For this review, take the finished solid that the model builds, in its own axes (mm). Face numbers are marked on the shaded views. A direction names the side the tool comes from. Give positions to 0.01 mm unless a question says otherwise; leave off trailing zeros. Write each loop counter-clockwise with the first axis right and the second up, starting at its lowest first coordinate (ties: lowest second). Pieces come first, ordered by that corner, then holes. Notation, with made-up numbers: M -26.75,-36.5 L 30.25,-36.5 A23 cw 30.25,-21.5 Z; hole C 26,78.5 d4. An arc over 180 degrees is marked long. One line per item, written item: value. Start each with the question number.
Item 1: Tool access review of the marked faces 1, 2 and 3: name each direction out of +Z, -Z, +X, -X, +Y, -Y from which nothing blocks a thin tool from reaching the whole face with its end or side.
Item 2: Mouldability with a two-part tool opening along X and no side actions: class the marked faces 4, 5 and 6 as released by +X, released by -X, zero draft, split by the parting line, or undercut.
Item 3: Clearance check with flat-ended pins moving along their axes: pin 1 Ø1.1 at (x, y) = (0, -1) entering from -Z; pin 2 Ø3 at (y, z) = (-5, 1.5) entering from +X; pin 3 Ø2 at (x, y) = (0.5, -3.5) entering from +Z. State where each tip first meets the part, or that it passes through.
Item 4: To check wall thickness, follow probe 1 along Y at (x, z) = (0.2, 0.2); probe 2 along X at (y, z) = (-11.25, -0.75); probe 3 along Y at (x, z) = (-1.4, -0.15). State the ranges of each line that lie inside material, in increasing order.
Item 5: Consider section A-A, the plane x = 0. Write out the cut boundary in (y, z).
Item 6: Consider section B-B, the plane y = -2.75. Write out the cut boundary in (x, z).
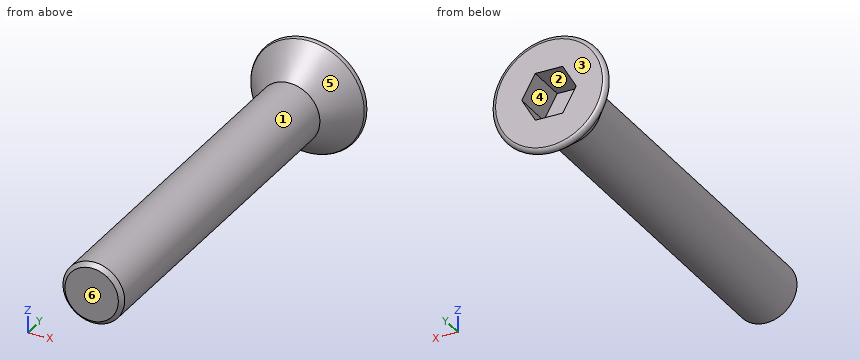
```python
from build123d import *

# Parameters (mm, degrees)
SKETCH_2_R          = 1.5
EXTRUDE_1_DEPTH     = 18
CUT_EXTRUDE_1_DEPTH = 2
CHAMFER_1_SIZE      = 0.2
FILLET_1_R          = 0.2


with BuildPart() as part:
    # 草图1 → 旋转1 (revolve)
    with BuildSketch(Plane.XY):
        Polygon((0, 0), (0, -2), (1.5, -2), (3, 0), align=None)
    revolve(axis=Axis((0, 0, 0), (0, -1, 0)))

    # 草图2 → 凸台-拉伸1 (add)
    with BuildSketch(Plane.XZ.offset(2)):
        Circle(SKETCH_2_R)
    extrude(amount=EXTRUDE_1_DEPTH)

    # 草图3 → 切除-拉伸1 (cut)
    with BuildSketch(Plane(origin=(0, 0, 0), x_dir=(1, 0, 0), z_dir=(0, 1, 0))):
        Polygon((-1.327905619, 0), (-0.66395281, -1.15), (0.66395281, -1.15), (1.327905619, 0), (0.66395281, 1.15), (-0.66395281, 1.15), align=None)
    extrude(amount=-CUT_EXTRUDE_1_DEPTH, mode=Mode.SUBTRACT)

    # 倒角1
    chamfer_1_edges = [part.edges().sort_by_distance(p)[0] for p in [
        (-1.5, -20, 0),
    ]]
    chamfer(chamfer_1_edges, length=CHAMFER_1_SIZE)

    # 圆角1
    fillet_1_edges = [part.edges().sort_by_distance(p)[0] for p in [
        (-3, 0, 0),
    ]]
    fillet(fillet_1_edges, radius=FILLET_1_R)


solid = part.part
```
Model answer:
1. face 1: -Y
1. face 2: +Y
1. face 3: +Z, -Z, +X, -X, +Y
2. face 4: undercut
2. face 5: split by the parting line
2. face 6: zero draft
3. pin 1: stops at z = -2.66
3. pin 2: stops at x = 1.5
3. pin 3: stops at z = 1.5
4. probe 1: y = -20 to -2
4. probe 2: x = -1.3 to 1.3
4. probe 3: y = -19.89 to 0
5. outline: M -20,-1.3 L -19.8,-1.5 L -2,-1.5 L -0.32,-2.76 A0.2 ccw 0,-2.6 L 0,-1.15 L -2,-1.15 L -2,1.15 L 0,1.15 L 0,2.6 A0.2 ccw -0.32,2.76 L -2,1.5 L -19.8,1.5 L -20,1.3 Z
6. outline: C 0,0 d3
